Autodesk Inventor part; units mm, degrees
ref_plane "YZ Plane" through (0, 0, 0) normal (1, 0, 0) x (0, 1, 0)
ref_plane "XZ Plane" through (0, 0, 0) normal (0, 1, 0) x (-1, 0, 0)
ref_plane "XY Plane" through (0, 0, 0) normal (0, 0, 1) x (1, 0, 0)
sketch "Sketch1" plane through (0, 0, 0) normal (0, 1, 0) x (-1, 0, 0)
  circle A0 centre (-0.1978, 0.0875) radius 15
  line L0 (0, 0) -> (25, 0)
  line L1 (0, 0) -> (-20.2254, -14.6946)
  line L2 (0, 0) -> (25, 0) construction
  line L3 (0, 0) -> (-20.2254, 14.6946)
  line L4 (0, 0) -> (25, 0) construction
  line L5 (25, 0) -> (14.5167, 0)
  line L6 (25, 0) -> (14.481, 0)
  line L7 (25, 2) -> (20, 2)
  line L8 (20, 2) -> (20, -2)
  line L9 (20, -2) -> (25, -2)
  line L10 (20, -2) -> (20, -3)
  line L11 (20, 2) -> (20, 3)
  line L12 (25, -2) -> (25, 2)
  line L13 (20, 3) -> (14.5167, 3)
  line L14 (20, -3) -> (14.481, -3)
  line L15 (-21.401, 13.0766) -> (-17.3559, 10.1377)
  line L16 (-17.3559, 10.1377) -> (-17.9437, 9.3287)
  line L17 (-19.0499, 16.3127) -> (-15.0048, 13.3737)
  line L18 (-15.0048, 13.3737) -> (-14.417, 14.1828)
  line L19 (-19.0499, 16.3127) -> (-21.401, 13.0766)
  line L20 (-17.9437, 9.3287) -> (-13.832, 6.3413)
  line L21 (-14.417, 14.1828) -> (-10.2902, 11.1845)
  line L22 (-19.0499, -16.3127) -> (-15.0048, -13.3737)
  line L23 (-15.0048, -13.3737) -> (-14.417, -14.1828)
  line L24 (-17.9437, -9.3287) -> (-17.3559, -10.1377)
  line L25 (-17.3559, -10.1377) -> (-21.401, -13.0766)
  line L26 (-19.0499, -16.3127) -> (-21.401, -13.0766)
  line L27 (-14.417, -14.1828) -> (-10.1826, -11.1063)
  line L28 (-17.9437, -9.3287) -> (-13.7712, -6.2971)
  line L29 (-17.9437, -9.3287) -> (-12.7862, -9.3287) construction
  point P0 (22.9129, 10)
  point P1 (-9.5074, 11.849)
  point P2 (-14.229, 5.3909)
  point P3 (-14.2604, -5.1319)
  point P4 (-9.5775, -11.6181)
  point P5 (14.2709, 4.0444)
  point P6 (14.247, -3.9556)
  dimension "d87" = 25
  dimension "d88" = 25
  dimension "d89" = 144
  dimension "d90" = 25
  dimension "d91" = 144
  dimension "d146" = 5
  dimension "d147" = 4
  dimension "d149" = 5
  dimension "d151" = 5
  dimension "d153" = 5
  dimension "d154" = 1
  dimension "d155" = 36
extrude "Extrusion1" add sketch "Sketch1" along normal blind 8
sketch "Sketch8" plane through (0, 8, 0) normal (0, 1, 0) x (1, 0, 0)
  circle A0 centre (0, 0) radius 4
  dimension "d80" = 8
extrude "Extrusion8" cut sketch "Sketch8" against normal blind 10
sketch "Sketch28" plane through (19.0499, 0, -16.3127) normal (0.809, 0, -0.5878) x (-0.5878, 0, -0.809)
  line L0 (-4, 8) -> (0, 8)
  line L1 (-2, 8) -> (-2, 0)
  line L2 (-2, 0) -> (-1, 0)
  line L3 (-4, 0) -> (0, 0)
  line L4 (-1, 0) -> (-1, 8)
  line L5 (-1, 8) -> (-3, 8)
  line L6 (-3, 8) -> (-3, 0)
  line L7 (-3, 0) -> (-1, 0)
  point P0 (-3, 8)
  point P1 (-3, 0)
  point P2 (-1, 8)
  dimension "d156" = 1
  dimension "d157" = 2
extrude "Extrusion26" cut sketch "Sketch28" against normal blind 8
sketch "Sketch29" plane through (21.401, 0, 13.0766) normal (0.809, 0, 0.5878) x (0.5878, 0, -0.809)
  line L0 (-4, 8) -> (0, 8)
  line L1 (-2, 0) -> (-1, 0)
  line L2 (-1, 0) -> (-1, 8)
  line L3 (-1, 8) -> (-2, 8)
  line L4 (-2, 8) -> (-2, 0)
  line L5 (-4, 0) -> (0, 0)
  line L6 (-1, 8) -> (-3, 8)
  line L7 (-3, 8) -> (-3, 0)
  line L8 (-3, 0) -> (-1, 0)
  line L9 (-1, 0) -> (-1, 8)
  point P0 (-3, 8)
  dimension "d160" = 1
  dimension "d161" = 2
extrude "Extrusion27" cut sketch "Sketch29" against normal blind 8
sketch "Sketch30" plane through (-25, 0, -2) normal (-1, 0, 0) x (0, 0, 1)
  line L0 (8.3413, 8) -> (-4.2971, 8)
  line L1 (2, 0) -> (3, 0)
  line L2 (3, 0) -> (3, 8)
  line L3 (3, 8) -> (2, 8)
  line L4 (2, 8) -> (2, 0)
  line L5 (8.3413, 0) -> (-4.2971, 0)
  line L6 (2, 8) -> (1, 8)
  line L7 (1, 8) -> (1, 0)
  line L8 (1, 0) -> (2, 0)
  line L9 (2, 0) -> (2, 8)
  dimension "d164" = 1
  dimension "d165" = 1
extrude "Extrusion28" cut sketch "Sketch30" against normal blind 8
sketch "Sketch31" plane through (-25, 0, 2) normal (0, 0, 1) x (1, 0, 0)
  line L0 (5, 8) -> (0, 8)
  line L1 (0, 8) -> (4.994, 0)
  line L2 (0, 0) -> (8, 0)
  circle A0 centre (2.497, 4) radius 1.5
  point P0 (25, 0)
  dimension "d168" = 3
sketch "Sketch32" plane through (17.3559, 0, 10.1377) normal (0.5878, 0, -0.809) x (-0.809, 0, -0.5878)
  line L0 (-5, 0) -> (0, 0)
  line L1 (3, 8) -> (-5, 8)
  line L2 (0, 0) -> (-5, 8)
  circle A0 centre (-2.5, 4) radius 1.5
  point P0 (20, 0)
  dimension "d169" = 3
sketch "Sketch33" plane through (15.0048, 0, -13.3737) normal (-0.5878, 0, -0.809) x (-0.809, 0, 0.5878)
  line L0 (-5, 8) -> (0, 8)
  line L1 (0, 0) -> (0, 8)
  line L2 (-5, 8) -> (0, 0)
  circle A0 centre (-2.5, 4) radius 1.5
  point P0 (20, 0)
  dimension "d170" = 3
extrude "Extrusion29" cut sketch "Sketch33" against normal blind 8 contours A0 L2 | L2 A0
extrude "Extrusion30" cut sketch "Sketch32" against normal blind 8
extrude "Extrusion31" cut sketch "Sketch31" against normal blind 8
properties part number "actuatorLink"
For this review, take the finished solid that the model builds, in its own axes (mm). A direction names the side the tool comes from. Round coordinates to 2 decimals unless told otherwise and drop trailing zeros. Write each loop counter-clockwise with the first axis right and the second up, starting at its lowest first coordinate (ties: lowest second). Pieces come first, ordered by that corner, then holes. Notation, with made-up numbers: (81.5, 16.25) -> (117.5, 16.25) arc R19 cw to (117.5, 42.25) -> close; hole circle Ø11 at (43.5, 44). An arc over 180 degrees is marked (long way). Put each result on its own line as item: value.
Q1. Consider section B-B on x = 0. State the section outline as (y, z) points, and give its area (3 significant figures).
Determined:
outline: (0, -14.91) -> (8, -14.91) -> (8, -4) -> (0, -4) -> close; (0, 4) -> (8, 4) -> (8, 15.09) -> (0, 15.09) -> close
area: 176 mm^2
Q2. Consider section A-A on z = 0. State the section outline as (x, y) points, and give its area (3 significant figures).
Determined:
outline: (-17, 0) -> (-4, 0) -> (-4, 8) -> (-17, 8) -> close; (4, 0) -> (15.2, 0) -> (15.2, 8) -> (4, 8) -> close
area: 194 mm^2
Q3. Consider section C-C on y = 4. Give the number of separate pieces and of enclosed holes in the cut face, and give its area (3 significant figures).
Determined:
separate pieces: 7
enclosed holes: 1
area: 742 mm^2
Q4. To check wall thickness, follow L1, parallel to Z at x = 0, y = 5.5; L2, parallel to X at y = 4, z = 1.75; L3, parallel to Z at x = 18, y = 1. State the ranges of each line that lie inside material, in increasing order. Write a range as [from, to].
Determined:
L1: z = [-14.91, -4], [4, 15.09]
L2: x = [-25, -24], [-21, -3.6], [3.6, 15.11]
L3: z = [-15.55, -14.31], [-11.84, -10.61], [10.61, 11.84], [14.31, 15.55]
Q5. Clearance check with flat-ended pins moving along their axes: pin 1 Ø2 at (y, z) = (6.5, -2.5) entering from +X; pin 2 Ø3.5 at (x, y) = (-22.503, 4) entering from -Z; pin 3 Ø13 at (x, z) = (0, 0) entering from -Y; pin 4 Ø1.5 at (y, z) = (3, -8.5) entering from +X. State where each tip first meets the part, or that it passes through.
Determined:
pin 1: stops at x = 15.11
pin 2: stops at z = -2
pin 3: stops at y = 0
pin 4: stops at x = 17.84
Q6. Machinability: for faces 1 (the flat face through (-20, 4, -1)), 2 (the flat face through (18.002, 3.944, -10.607)), 3 (the flat face through (12.329, 3.944, -12.666)), 4 (the flat face through (-20.8, 3.9, -2)), which of the approach directions +Z, -Z, +X, -X, +Y, -Y give a long, thin tool a straight path to every point of the face, cutting with its end or side? Answer none if there is none.
Determined:
face 1: -X, +Y, -Y
face 2: +X, +Y, -Y
face 3: -Z, +Y, -Y
face 4: -Z, -X, +Y, -Y
Q7. The part is to be moulded in two halves that separate along Y. For faces 5 (the flat face through (15.887, 3.944, -7.834)), 6 (the cylindrical face through (20.3, 4.07, 12.89)), 7 (the flat face through (-1.5, 0, 3.9)), 8 (the cylindrical face through (16.16, 4.45, -13.6)), say which applies: released by +Y, released by -Y, zero draft, split by the parting line, or undercut.
Determined:
face 5: zero draft
face 6: undercut
face 7: released by -Y
face 8: undercut
